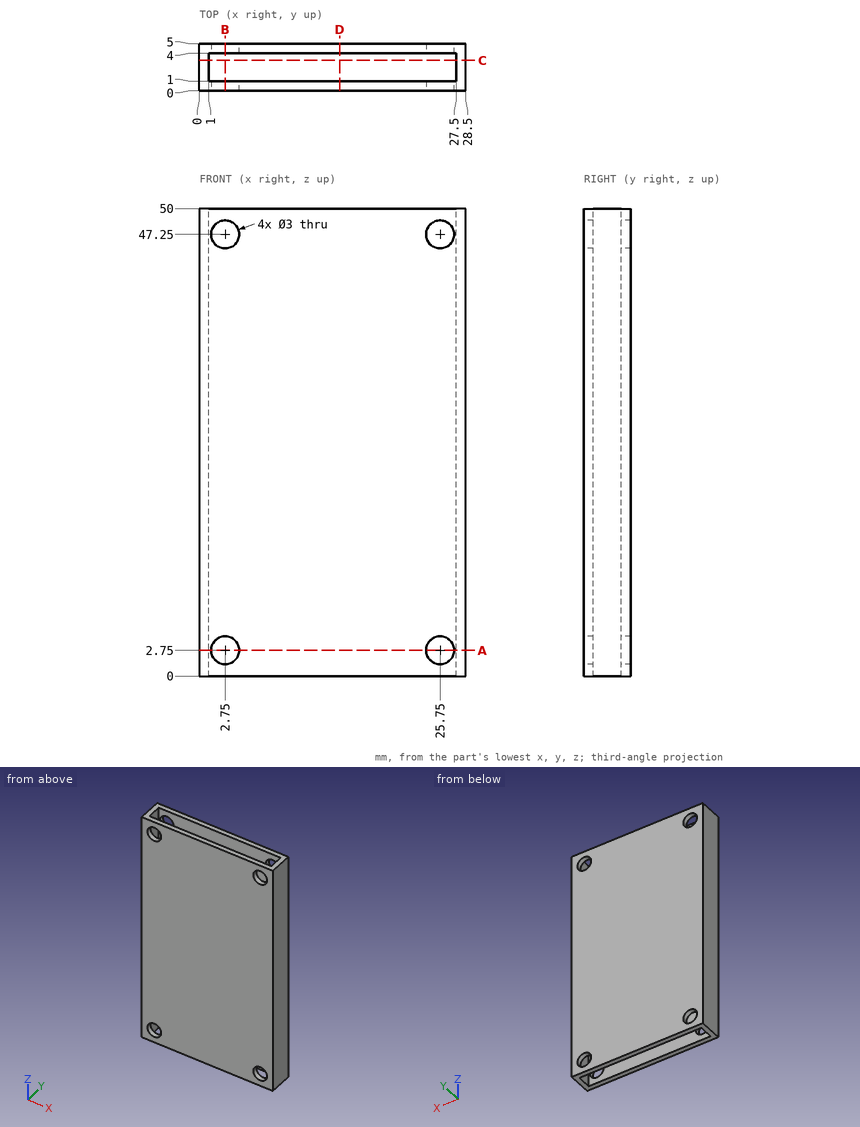
Can you work these out from the drawing? Everything is in mm from the part's minimum corner. Give positions to 0.01 mm unless a question says otherwise; leave off trailing zeros. Write each loop counter-clockwise with the first axis right and the second up, starting at its lowest first coordinate (ties: lowest second). Pieces come first, ordered by that corner, then holes. Notation, with made-up numbers: (46, 23) -> (78, 23) arc R16 cw to (78, 32) -> close; hole circle Ø7 at (1, -11.5). An arc over 180 degrees is marked (long way). Write each question's results on one line, items separated by ' | '. Start each with the question number.
Q1. Suppose I cut it at C-C, the plane y = 3.25. List the corners of the cut face in (x, z) for me, and give its area (3 significant figures).
Q2. I'm going to push flat-ended pins straight in: pin 1 Ø1.8 at (x, z) = (25.75, 47.25) entering from -Y; pin 2 Ø8 at (x, z) = (14.5, 22) entering from -Y. Where does each tip first touch, or does it pass through?
Q3. Suppose I cut it at A-A, the plane z = 2.75. List the corners of the cut face in (x, y) for me, and give its area (3 significant figures).
Q4. Suppose I cut it at B-B, the plane x = 2.75. List the corners of the cut face in (y, z) for me, and give its area (3 significant figures).
Q5. Suppose I cut it at D-D, the plane x = 15. List the corners of the cut face in (y, z) for me.
Q6. I need wall thicknesses on probe 1 along Z at (x, y) = (25.75, 4.5); probe 2 along X at (y, z) = (0.3, 47.25); probe 3 along X at (y, z) = (3.85, 5.5). Which ranges of each line are inside material? Lowest first, please.
Outcome:
1) outline: (0, 0) -> (1, 0) -> (1, 50) -> (0, 50) -> close; (27.5, 0) -> (28.5, 0) -> (28.5, 50) -> (27.5, 50) -> close | area: 100 mm2
2) pin 1: through | pin 2: y = 0
3) outline: (0, 0) -> (1.25, 0) -> (1.25, 1) -> (1, 1) -> (1, 4) -> (1.25, 4) -> (1.25, 5) -> (0, 5) -> close; (4.25, 0) -> (24.25, 0) -> (24.25, 1) -> (4.25, 1) -> close; (4.25, 4) -> (24.25, 4) -> (24.25, 5) -> (4.25, 5) -> close; (27.25, 0) -> (28.5, 0) -> (28.5, 5) -> (27.25, 5) -> (27.25, 4) -> (27.5, 4) -> (27.5, 1) -> (27.25, 1) -> close | area: 51.0 mm2
4) outline: (0, 0) -> (1, 0) -> (1, 1.25) -> (0, 1.25) -> close; (0, 4.25) -> (1, 4.25) -> (1, 45.75) -> (0, 45.75) -> close; (0, 48.75) -> (1, 48.75) -> (1, 50) -> (0, 50) -> close; (4, 0) -> (5, 0) -> (5, 1.25) -> (4, 1.25) -> close; (4, 4.25) -> (5, 4.25) -> (5, 45.75) -> (4, 45.75) -> close; (4, 48.75) -> (5, 48.75) -> (5, 50) -> (4, 50) -> close | area: 88.0 mm2
5) outline: (0, 0) -> (1, 0) -> (1, 50) -> (0, 50) -> close; (4, 0) -> (5, 0) -> (5, 50) -> (4, 50) -> close
6) probe 1: 0 to 1.25, 4.25 to 45.75, 48.75 to 50 | probe 2: 0 to 1.25, 4.25 to 24.25, 27.25 to 28.5 | probe 3: 0 to 1, 27.5 to 28.5
